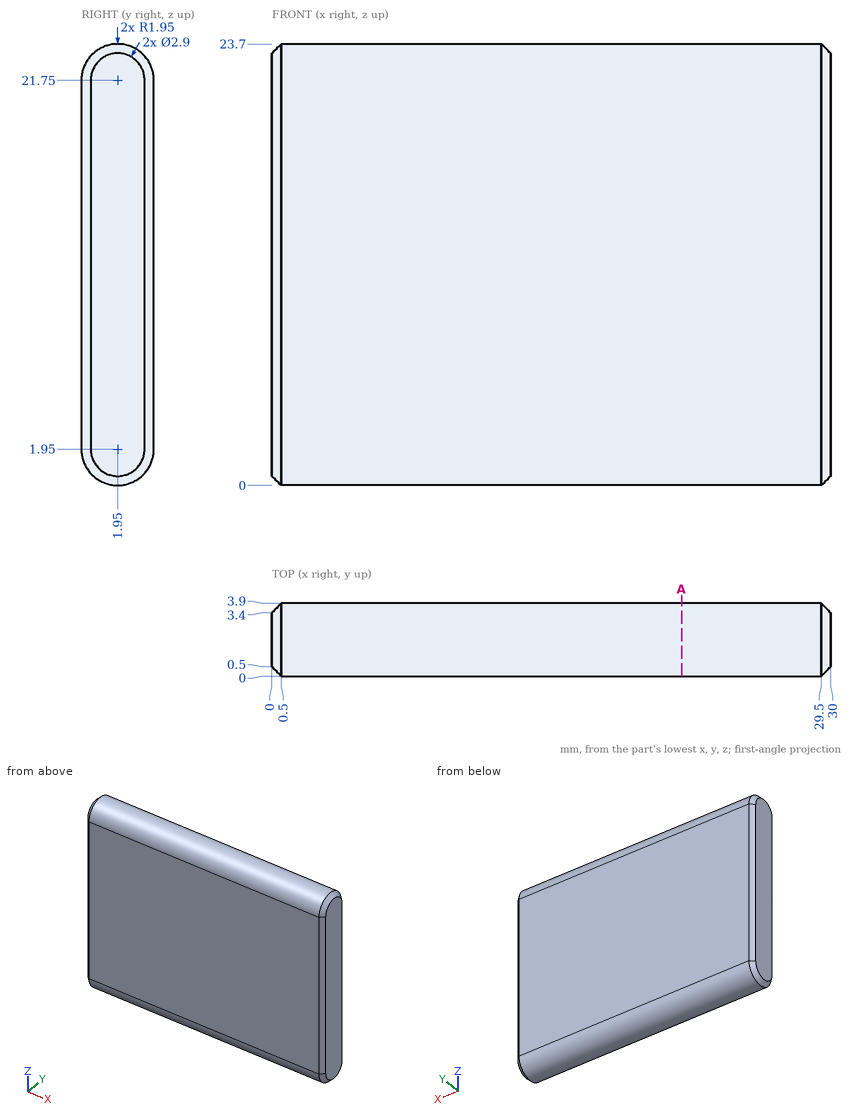
Part print with two shaded views. Sizes in mm from the minimum x, y, z corner. Give positions to 0.01 mm unless a question says otherwise; leave off trailing zeros. Loops run counter-clockwise (first coordinate to the right, second up) from the corner with the lowest first, then second, coordinate; pieces in that order, holes last. Notation, with made-up numbers: (-16, 48.25) -> (32, 48.25) arc R24 ccw to (32, 63.25) -> close; hole circle Ø7 at (27, 0). An arc over 180 degrees is marked (long way). One line per question, with ' | ' between items.
Q1. Drill centre lines: line 1 along Z through (x, y) = (18.5, 1.8); line 2 along X through (y, z) = (3.05, 1); line 3 along Z through (x, y) = (12, 0.25). Where is each one in solid material? Low to high. Write a range as [from, to].
Filled sheet:
line 1: z = [0.01, 23.69] | line 2: x = [0, 30] | line 3: z = [0.99, 22.71]
Q2. Drop a flat-ended pin along its axis: pin 1 (12 mm diameter, centred on x = 6.5, z = 17.5, fed in from -Y). Give the stop position or say it passes through.
Filled sheet:
pin 1: stops at y = 0
Q3. Cut at A-A, the plane x = 22. Write the cut outline in (y, z).
Filled sheet:
outline: (0, 1.95) arc R1.95 ccw to (3.9, 1.95) -> (3.9, 21.75) arc R1.95 ccw to (0, 21.75) -> close
